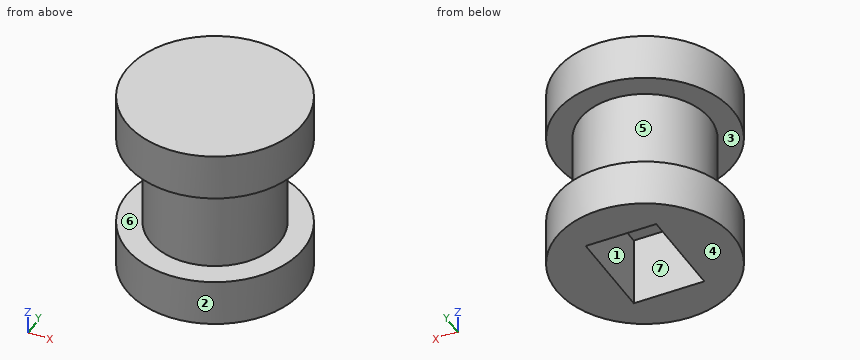
from build123d import *

# Parameters (mm, degrees)
SKETCH1_R           = 4.7625
BOSS_EXTRUDE1_DEPTH = 5.08
SKETCH4_W           = 3.81
SKETCH4_H           = 5.08
CUT_EXTRUDE1_DEPTH  = 3.81
SKETCH8_W           = 5.08
SKETCH8_H           = 2.54


with BuildPart() as part:
    # Sketch1 → Boss-Extrude1 (new body, symmetric)
    with BuildSketch(Plane.XY):
        Circle(SKETCH1_R)
    extrude(amount=BOSS_EXTRUDE1_DEPTH, both=True)

    # Sketch4 → Cut-Extrude1 (cut)
    with BuildSketch(Plane(origin=(0, 0, -5.08), x_dir=(-1, 0, 0), z_dir=(0, 0, -1))):
        Rectangle(SKETCH4_W, SKETCH4_H)
    extrude(amount=-CUT_EXTRUDE1_DEPTH, mode=Mode.SUBTRACT)

    # Sketch8 → Cut-Revolve1 (revolve, cut)
    with BuildSketch(Plane(origin=(0, 0, 0), x_dir=(0, 0, -1), z_dir=(1, 0, 0)), mode=Mode.PRIVATE) as cut_revolve1_sk:
        with Locations((0, 4.7625)):
            Rectangle(SKETCH8_W, SKETCH8_H)
    revolve(cut_revolve1_sk.sketch.rotate(Axis((0, 0, 0), (0, 0, -1)), 90), axis=Axis((0, 0, 0), (0, 0, -1)), mode=Mode.SUBTRACT)  # turned: the seam where the file's is


solid = part.part
Could you check a few things on this model? Use its own coordinates, in mm. Face numbers are marked on the shaded views. A direction names the side the tool comes from. Coordinates: 2 decimals unless noted, no trailing zeros. Loops run counter-clockwise (first coordinate to the right, second up) from the corner with the lowest first, then second, coordinate; pieces in that order, holes last. Notation, with made-up numbers: (-8, 47) -> (-1, 47) arc R11 cw to (-1, 57) -> close; hole circle Ø2 at (6, 45). An arc over 180 degrees is marked (long way). Answer in a Markdown table with one row per item.
(1) If I drill on probe 1 along Z at (x, y) = (1.5, -3.25); probe 2 along Z at (x, y) = (1.5, 1.75); probe 3 along X at (y, z) = (2, -3) (3 decimals), over which ranges is the centre line in solid material (lowest first)?
Results found:
| item | result |
|---|---|
| probe 1 | z = -5.08 to -2.54, 2.54 to 5.08 |
| probe 2 | z = -1.27 to 5.08 |
| probe 3 | x = -4.322 to -1.905, 1.905 to 4.322 |
(2) For the marked faces 1, 2 and 3, which set-ups out of +Z, -Z, +X, -X, +Y, -Y let a thin tool reach every point of the face, with its end or its side?
Results found:
| item | result |
|---|---|
| face 1 | -Z |
| face 2 | +Z, -Z |
| face 3 | none |
(3) Imagine slicing it at D-D (z = 2.75). List the corners of the cut face in (x, y) for me (1 decimal), plus the area to 3 significant figures.
Results found:
| item | result |
|---|---|
| outline | circle Ø9.5 at (0, 0) |
| area | 71.3 mm^2 |
(4) Imagine slicing it at C-C (x = 0). List the corners of the cut face in (y, z) for me.
Results found:
| item | result |
|---|---|
| outline | (-4.76, -5.08) -> (-2.54, -5.08) -> (-2.54, -1.27) -> (2.54, -1.27) -> (2.54, -5.08) -> (4.76, -5.08) -> (4.76, -2.54) -> (3.49, -2.54) -> (3.49, 2.54) -> (4.76, 2.54) -> (4.76, 5.08) -> (-4.76, 5.08) -> (-4.76, 2.54) -> (-3.49, 2.54) -> (-3.49, -2.54) -> (-4.76, -2.54) -> close |
(5) Imagine slicing it at A-A (x = 3.75). List the corners of the cut face in (y, z) for me.
Results found:
| item | result |
|---|---|
| outline | (-2.94, -5.08) -> (2.94, -5.08) -> (2.94, -2.54) -> (-2.94, -2.54) -> close; (-2.94, 2.54) -> (2.94, 2.54) -> (2.94, 5.08) -> (-2.94, 5.08) -> close |
(6) Thinking about a two-plate mould opening in Z: for the marked faces 4, 5, 6 and 7, which applies, released by +Z, released by -Z, zero draft, split by the parting line, or undercut?
Results found:
| item | result |
|---|---|
| face 4 | released by -Z |
| face 5 | undercut |
| face 6 | undercut |
| face 7 | zero draft |
(7) Will these pins go through, and if not, where does the flat tip stop? pin 1 Ø3 at (x, y) = (0.5, -0.5) entering from -Z; pin 2 Ø1 at (x, z) = (-2.5, -3.5) entering from -Y; pin 3 Ø1.1 at (y, z) = (1, -3.5) entering from -X; pin 4 Ø1 at (x, z) = (-1.5, -2) entering from -Y.
Results found:
| item | result |
|---|---|
| pin 1 | stops at z = -5.08 |
| pin 2 | stops at y = -4.32 |
| pin 3 | stops at x = -4.74 |
| pin 4 | stops at y = -3.35 |
(8) Imagine slicing it at B-B (y = 0). List the corners of the cut face in (x, z) for me (1 decimal), plus the area to 3 significant figures.
Results found:
| item | result |
|---|---|
| outline | (-4.8, -5.1) -> (-1.9, -5.1) -> (-1.9, -1.3) -> (1.9, -1.3) -> (1.9, -5.1) -> (4.8, -5.1) -> (4.8, -2.5) -> (3.5, -2.5) -> (3.5, 2.5) -> (4.8, 2.5) -> (4.8, 5.1) -> (-4.8, 5.1) -> (-4.8, 2.5) -> (-3.5, 2.5) -> (-3.5, -2.5) -> (-4.8, -2.5) -> close |
| area | 69.4 mm^2 |
